Here's how the part is built. I have some questions about the finished solid (model axes, mm). Give positions to 0.01 mm unless a question says otherwise; leave off trailing zeros. Write each loop counter-clockwise with the first axis right and the second up, starting at its lowest first coordinate (ties: lowest second). Pieces come first, ordered by that corner, then holes. Notation, with made-up numbers: (28.5, 88.25) -> (69.5, 88.25) arc R18 ccw to (69.5, 98.25) -> close; hole circle Ø5 at (20, 59.25). An arc over 180 degrees is marked (long way). Answer as CSV lines item,"result". Start each with the question number.
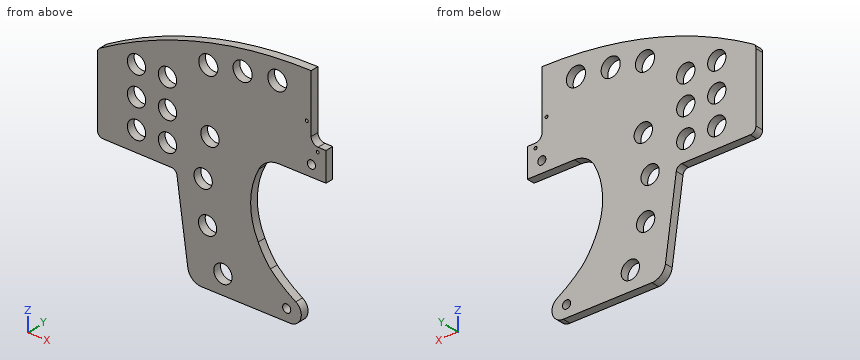
from build123d import *

# Parameters (mm, degrees)
MIRROREDSKETCH_R      = 3.5
PAD022_DEPTH          = 7
MIRROREDSKETCH001_R   = 1.25
POCKET031_DEPTH       = 37.001
MIRROREDSKETCH002_R   = 7.9
MIRROREDSKETCH002_R_2 = 8.25
POCKET032_DEPTH       = 7.001


with BuildPart() as part:
    # MirroredSketch → Pad022 (new body)
    with BuildSketch(Plane.XZ):
        with BuildLine():
            Line((-272.354121, 37.429427), (-272.343757, -21.795436))
            ThreePointArc((-272.343757, -21.795436), (-270.889508, -25.319746), (-267.373614, -26.794228))
            Line((-267.373614, -26.794228), (-208.288633, -27.144182))
            ThreePointArc((-203.514267, -31.323983), (-205.122941, -28.344833), (-208.288633, -27.144182))
            Line((-203.514267, -31.323983), (-194.118707, -98.712795))
            ThreePointArc((-194.118707, -98.712795), (-190.168756, -106.001984), (-182.403958, -108.907549))
            Line((-182.403958, -108.907549), (-105.81311, -108.907549))
            ThreePointArc((-105.81311, -108.907549), (-96.416366, -101.749846), (-100.820682, -90.789302))
            ThreePointArc((-122.731662, -73.595005), (-112.325474, -82.892139), (-100.820682, -90.789302))
            ThreePointArc((-133.286541, -56.888144), (-128.564005, -65.592146), (-122.731662, -73.595005))
            ThreePointArc((-132.652743, -0.740873), (-139.8492, -28.736851), (-133.286541, -56.888144))
            ThreePointArc((-115.533318, 9.507899), (-125.509691, 6.749885), (-132.652743, -0.740873))
            Line((-74.738136, 9.507899), (-115.533318, 9.507899))
            Line((-74.738136, 34.5363), (-74.738136, 9.507899))
            Line((-74.738136, 34.5363), (-81.548261, 34.57921))
            ThreePointArc((-87.538437, 40.605923), (-85.785771, 36.357677), (-81.548261, 34.57921))
            Line((-87.538437, 40.605923), (-87.54951, 90.990038))
            ThreePointArc((-87.54951, 90.990038), (-182.019209, 78.593902), (-269.883601, 41.742351))
            ThreePointArc((-269.883601, 41.742351), (-271.692728, 39.91461), (-272.354121, 37.429427))
        make_face()
        with Locations((-87.265671, 19.281441)):
            Circle(MIRROREDSKETCH_R, mode=Mode.SUBTRACT)
        with Locations((-108.660279, -98.693397)):
            Circle(MIRROREDSKETCH_R, mode=Mode.SUBTRACT)
    extrude(amount=PAD022_DEPTH)

    # MirroredSketch001 → Pocket031 (cut, through all)
    with BuildSketch(Plane.XZ.offset(37)):
        with Locations((-81.894829, 30.717421)):
            Circle(MIRROREDSKETCH001_R)
        with Locations((-91.346397, 51.206974)):
            Circle(MIRROREDSKETCH001_R)
    extrude(amount=-POCKET031_DEPTH, mode=Mode.SUBTRACT)

    # MirroredSketch002 → Pocket032 (cut, through all)
    with BuildSketch(Plane.XZ.offset(7)):
        with Locations((-211.699159, 15.680032)):
            Circle(MIRROREDSKETCH002_R)
        with Locations((-211.699159, -9.396934)):
            Circle(MIRROREDSKETCH002_R)
        with Locations((-238.46666, 15.680032)):
            Circle(MIRROREDSKETCH002_R)
        with Locations((-238.46666, -9.396934)):
            Circle(MIRROREDSKETCH002_R)
        with Locations((-211.699159, 40.756998)):
            Circle(MIRROREDSKETCH002_R)
        with Locations((-238.46666, 40.756998)):
            Circle(MIRROREDSKETCH002_R)
        with Locations((-180.85994, -25.593019)):
            Circle(MIRROREDSKETCH002_R)
        with Locations((-177.027703, -60.155267)):
            Circle(MIRROREDSKETCH002_R)
        with Locations((-163.777795, -92.306084)):
            Circle(MIRROREDSKETCH002_R)
        with Locations((-174.975, 8.679456)):
            Circle(MIRROREDSKETCH002_R)
        with Locations((-116.788777, 72.751051)):
            Circle(MIRROREDSKETCH002_R_2)
        with Locations((-146.796527, 68.916422)):
            Circle(MIRROREDSKETCH002_R_2)
        with Locations((-176.435989, 62.860703)):
            Circle(MIRROREDSKETCH002_R_2)
    extrude(amount=-POCKET032_DEPTH, mode=Mode.SUBTRACT)


solid = part.part
Item 1: If I drill on line 1 (Z direction, x = -177.5, y = -6); line 2 (Z direction, x = -175, y = -3.5); line 3 (Z direction, x = -210, y = -3), over which ranges is the centre line in solid material (lowest first)? Write a range as [from, to].
Item 2: If we section it at B-B (z = 46): Please give me the cut outline in (x, y).
Item 3: If we section it at C-C (y = -4.25): State how many separate pieces and enclosed holes the cut face has, and give its area (3 significant figures).
Item 4: If we section it at A-A (x = -164.5): Please give me the cut outline in (y, z).
Item 5: I'm going to push flat-ended pins straight in: pin 1 (2 mm diameter, centred on x = -182, y = -1.5, fed in from +Z); pin 2 (1.5 mm diameter, centred on x = -135.5, y = -1, fed in from +Z); pin 3 (3 mm diameter, centred on y = -1, z = -48.5, fed in from +X). Where does each tip first touch, or does it pass through?
Item 6: If we section it at D-D (x = -129): Please give me the cut outline in (y, z).
Final values:
1,line 1,"[-108.91, -68.04], [-52.27, -32.74], [-18.44, 1.19], [16.17, 54.68], [71.04, 79.78]"
1,line 2,"[-108.91, -67.79], [-52.52, -30.89], [-20.29, 0.78], [16.58, 54.74], [70.98, 80.41]"
1,line 3,"[-27.13, -17.11], [-1.68, 7.96], [23.4, 33.04], [48.47, 69.79]"
2,outline,"(-262.42, -7) -> (-244.38, -7) -> (-244.38, 0) -> (-262.42, 0) -> close; (-232.56, -7) -> (-217.61, -7) -> (-217.61, 0) -> (-232.56, 0) -> close; (-205.79, -7) -> (-87.54, -7) -> (-87.54, 0) -> (-205.79, 0) -> close"
3,separate pieces,"1"
3,enclosed holes,"17"
3,area,"21,000 mm2"
4,outline,"(-7, -108.91) -> (0, -108.91) -> (0, -100.17) -> (-7, -100.17) -> close; (-7, -84.44) -> (0, -84.44) -> (0, 82.86) -> (-7, 82.86) -> close"
5,pin 1,"z = 78.87"
5,pin 2,"z = 88"
5,pin 3,"x = -136.26"
6,outline,"(-7, -108.91) -> (0, -108.91) -> (0, -64.89) -> (-7, -64.89) -> close; (-7, 4.08) -> (0, 4.08) -> (0, 88.7) -> (-7, 88.7) -> close"
